from build123d import *


with BuildPart() as f1:
    # F0 (on Top) → F1 (revolve)
    with BuildSketch(Plane.XY):
        Polygon((0, 10), (0, 1), (2, 1), (2, 4), (2, 10), align=None)
        Polygon((2, 4), (2, 1), (5, 1), (5, 3.5), (4.5, 4), align=None)
    revolve(axis=Axis((5.453455, 0, 0), (1, 0, 0)))


solid = f1.part
Can you work these out from the model? Positions are in its coordinate system, mm. A direction names the side the tool comes from. Round coordinates to 2 decimals unless told otherwise and drop trailing zeros. Loops run counter-clockwise (first coordinate to the right, second up) from the corner with the lowest first, then second, coordinate; pieces in that order, holes last. Notation, with made-up numbers: (33.25, 2) - (44.25, 2) arc R25 cw to (44.25, 35) - close; hole circle Ø10 at (68.5, -26). An arc over 180 degrees is marked (long way). Write item = value, one per line. Start each with the question number.
(1) If I drill on probe 1 along Z at (x, y) = (3.2, 0); probe 2 along X at (y, z) = (-7, -2); probe 3 along Y at (x, z) = (2.6, 3), over which ranges is the centre line in solid material (lowest first)? Write a range as [from, to].
(2) If we mould it in two halves opening along Y, with no side actions, what happens to faces 3 (the face through (3, 0, -1)), 4 (the face through (3.232, -0.867, -3.905)), 5 (the face through (5, -1, -1))? For each: released by +Y, released by -Y, zero draft, split by the parting line, or undercut.
(3) If we section it at D-D (x = 1.15): Please give me the cut outline in (y, z).
(4) If we section it at A-A (y = 0): Please give me the cut outline in (x, z).
(5) For faces 1 (the face through (0.99, -2.17, -9.76)), 2 (the face through (2, -4.3, 0.1)), which set-ups out of +Z, -Z, +X, -X, +Y, -Y let a thin tool reach every point of the face, with its end or its side?
(6) If we section it at C-C (x = 3.85): Please give me the cut outline in (y, z), and give its area (3 significant figures).
Ans:
q1.probe_1 = [-4, -1], [1, 4]
q1.probe_2 = [0, 2]
q1.probe_3 = [-2.65, 2.65]
q2.face_3 = undercut
q2.face_4 = split by the parting line
q2.face_5 = zero draft
q3.outline = circle Ø20 at (0, 0); hole circle Ø2 at (0, 0)
q4.outline = (0, -10) - (2, -10) - (2, -4) - (4.5, -4) - (5, -3.5) - (5, -1) - (0, -1) - close; (0, 1) - (5, 1) - (5, 3.5) - (4.5, 4) - (2, 4) - (2, 10) - (0, 10) - close
q5.face_1 = +X, -X
q5.face_2 = +X
q6.outline = circle Ø8 at (0, 0); hole circle Ø2 at (0, 0)
q6.area = 47.1 mm²
